Could you check a few things on this model? Use its own coordinates, in mm. A direction names the side the tool comes from. Give positions to 0.01 mm unless a question says otherwise; leave off trailing zeros. Loops run counter-clockwise (first coordinate to the right, second up) from the corner with the lowest first, then second, coordinate; pieces in that order, holes last. Notation, with made-up numbers: (-8, 89.5) - (47, 89.5) arc R20 ccw to (47, 94.5) - close; hole circle Ø11 at (48.25, 30.5). An arc over 180 degrees is marked (long way). Write each question's results on one line, items separated by ' | '. Start each with the question number.
(1) Suppose I cut it at B-B (y = -17). Please give me the cut outline in (x, z).
(2) Suppose I cut it at D-D (y = -10.5). Please give me the cut outline in (x, z).
(3) Suppose I cut it at C-C (x = 27). Please give me the cut outline in (y, z).
(4) On a 3-axis mill with a long thin cutter (end or side, diameter ignored), from which of +Z, -Z, +X, -X, +Y, -Y can I reach the whole of each face in a straight line? I mean faces 1 (the face through (-2, -36.533, -2)), 2 (the face through (-2, -3.62, -2)), 3 (the face through (-31, -25, 9.166)), 4 (the face through (0, -20, -2)). Say none if no direction works.
(5) I need wall thicknesses on line 1 (X direction, y = -26, z = 0); line 2 (X direction, y = -40, z = 0); line 3 (Z direction, x = -50, y = -15). Which ranges of each line are inside material? Lowest first, please.
(6) For pin 1 (5 mm diameter, centred on x = 13.5, y = -48.5, fed in from -Z); pin 2 (10 mm diameter, centred on y = -48.5, z = 12.5, fed in from -X); pin 3 (1.5 mm diameter, centred on x = -6.5, z = 10, fed in from +Y); pin 4 (7 mm diameter, centred on x = -29, y = -20.5, fed in from +Z), each with a flat end and sliding along its axis, tell me the tip position at first contact or that it passes through.
(7) Suppose I cut it at A-A (z = 0). Please give me the cut outline in (x, y).
(8) If we mould it in two halves opening along X, with no side actions, what happens to faces 5 (the face through (-5.585, -6, 20)), 6 (the face through (-33, -6, 22.947)), 7 (the face through (-50.8, -25, -5))? For each: released by +X, released by -X, zero draft, split by the parting line, or undercut.
from build123d import *

# Parameters (mm, degrees)
F1_R     = 26.716265
F1_R_2   = 18.954544
F2_DEPTH = 63.5
F0_W     = 53.663762
F0_H     = 50.992716
F3_DEPTH = 12.7
F4_W     = 32.913139
F4_H     = 28.322212
F5_DEPTH = 50.8


with BuildPart() as f2:
    # F1 (on Front) → F2 (new body)
    with BuildSketch(Plane.XZ):
        with Locations((14.083703, 0)):
            Circle(F1_R)
        with Locations((14.083703, 0)):
            Circle(F1_R_2, mode=Mode.SUBTRACT)
    extrude(amount=F2_DEPTH)

    # F0 (on Front) → F3 (join)
    with BuildSketch(Plane.XZ):
        with Locations((-32.416797, -2.549635)):
            Rectangle(F0_W, F0_H)
    extrude(amount=F3_DEPTH)

    # F4 (on Right) → F5 (join)
    with BuildSketch(Plane.YZ):
        with Locations((-20.076167, -4.994778)):
            Rectangle(F4_W, F4_H)
    extrude(amount=-F5_DEPTH)


solid = f2.part
Output values:
1) outline: (-50.8, -19.16) - (-4.54, -19.16) arc R26.72 ccw (long way) to (-11.01, 9.17) - (-50.8, 9.17) - close; hole (-2.51, 9.17) - (0, 9.17) - (0, -12.69) arc R18.95 ccw (long way) to start
2) outline: (-59.25, -28.05) - (-5.58, -28.05) - (-5.58, -19.16) - (-4.54, -19.16) arc R26.72 ccw (long way) to (-5.58, 18.08) - (-5.58, 22.95) - (-59.25, 22.95) - close; hole (-2.51, 9.17) - (0, 9.17) - (0, -12.69) arc R18.95 ccw (long way) to start
3) outline: (-63.5, -23.39) - (0, -23.39) - (0, -13.87) - (-63.5, -13.87) - close; (-63.5, 13.87) - (0, 13.87) - (0, 23.39) - (-63.5, 23.39) - close
4) face 1: -Y | face 2: +Y | face 3: +Z, -X, -Y | face 4: +Y, -Y
5) line 1: -50.8 to 0, 33.04 to 40.8 | line 2: -12.63 to -4.87, 33.04 to 40.8 | line 3: -19.16 to 9.17
6) pin 1: z = -26.72 | pin 2: x = -11.56 | pin 3: y = 0 | pin 4: z = 9.17
7) outline: (-59.25, -12.7) - (-50.8, -12.7) - (-50.8, -36.53) - (-12.63, -36.53) - (-12.63, -63.5) - (-4.87, -63.5) - (-4.87, -36.53) - (0, -36.53) - (0, -3.62) - (-4.87, -3.62) - (-4.87, 0) - (-59.25, 0) - close; (33.04, -63.5) - (40.8, -63.5) - (40.8, 0) - (33.04, 0) - close
8) face 5: undercut | face 6: zero draft | face 7: released by -X
